```python
from build123d import *

# Parameters (mm, degrees)
F0_W           = 18.9992
F0_H           = 18.9992
F1_DEPTH       = 5.588
F2_R           = 3.175
F4_D           = 5.588
F4_CSINK_D     = 11.176
F4_CSINK_ANGLE = 82


with BuildPart() as f1:
    # F0 (on Front) → F1 (new body)
    with BuildSketch(Plane.XZ):
        with Locations((9.4996, 9.4996)):
            Rectangle(F0_W, F0_H)
    extrude(amount=F1_DEPTH)

    # F2
    f2_edges = [f1.edges().sort_by_distance(p)[0] for p in [
        (0, -2.794, 18.9992),
        (18.9992, -2.794, 18.9992),
        (18.9992, -2.794, 0),
        (0, -2.794, 0),
    ]]
    fillet(f2_edges, radius=F2_R)

    # F4 (through all)
    with Locations(Plane.XZ.offset(5.588)):
        with Locations((9.4996, 9.4996)):
            CounterSinkHole(F4_D / 2, F4_CSINK_D / 2, counter_sink_angle=F4_CSINK_ANGLE)


solid = f1.part
```
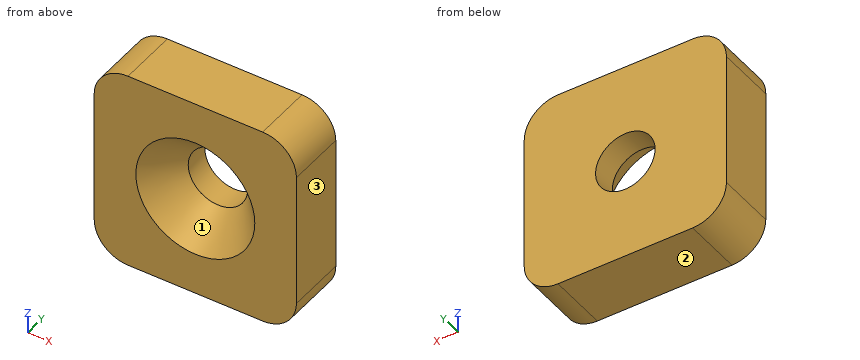
Model file for the job. Use its own axes, mm. Face numbers are marked on the shaded views. Round coordinates to 2 decimals unless told otherwise and drop trailing zeros. Write each loop counter-clockwise with the first axis right and the second up, starting at its lowest first coordinate (ties: lowest second). Pieces come first, ordered by that corner, then holes. Notation, with made-up numbers: M 45,-4 L 74,-4 A25 cw 74,21 Z; hole C 84.5,40.5 d4. An arc over 180 degrees is marked long. Put each result on its own line as item: value.
Item 1: Cut at C-C (z = 2). List the corners of the cut face in (x, y).
Responses:
outline: M 0.23,-5.59 L 18.77,-5.59 L 18.77,0 L 0.23,0 Z
Item 2: Cut at B-B (y = -1.85). List the corners of the cut face in (x, z) (3 decimals).
Responses:
outline: M 0,3.175 A3.175 ccw 3.175,0 L 15.824,0 A3.175 ccw 18.999,3.175 L 18.999,15.824 A3.175 ccw 15.824,18.999 L 3.175,18.999 A3.175 ccw 0,15.824 Z; hole C 9.5,9.5 d5.588
Item 3: Mould opens along Z. For the marked faces 1, 2 and 3 say: +Z half, -Z half, draft (parallel to the pull), parting line (faces both ways), or undercut.
Responses:
face 1: undercut
face 2: -Z half
face 3: draft
Item 4: Flat gauge pins, fed straight in: P1, Ø1, axis at x = 9.5, z = 4.5, coming from the -Y side; P2, Ø4.5, axis at x = 9.5, z = 9.5, coming from the -Y side. Where does each tip first touch, or does it go through?
Responses:
P1: y = -5.49
P2: through
Item 5: Probe L1, parallel to X at y = -2.95, z = 16; L2, parallel to X at y = -4.6, z = 10.75. List the from-to ranges inside material, lowest first. Write a range as from..to.
Responses:
L1: 0..18.99
L2: 0..4.94, 14.06..19
